```python
from build123d import *

# Parameters (mm, degrees)
BOSS_EXTRUDE1_DEPTH      = 76.2
BOSS_EXTRUDE1_DEPTH_BACK = 76.2
CUT_EXTRUDE1_DEPTH       = 136.619651209
CUT_EXTRUDE1_DEPTH_BACK  = 136.619651209
FILLET1_R                = 3.81
SKETCH14_R               = 2.032
CUT_EXTRUDE8_DEPTH       = 156.372005628
CUT_EXTRUDE9_DEPTH       = 136.355460931
CUT_EXTRUDE9_DEPTH_BACK  = 136.355460931
SKETCH15_W               = 96.731852598
SKETCH15_H               = 147.433285995
SKETCH15_W_2             = 126.258869859
SKETCH15_H_2             = 31.294033563
CUT_EXTRUDE10_DEPTH      = 112.88020808
CUT_EXTRUDE10_DEPTH_BACK = 112.88020808
SKETCH16_R               = 2.127


with BuildPart() as part:
    # Sketch1 → Boss-Extrude1 (new, two sides: drawn at the far end of the back side and taken through both)
    with BuildSketch(Plane.XY.offset(-BOSS_EXTRUDE1_DEPTH_BACK)):
        with BuildLine():
            Line((-6.335258536, -105.245804705), (-12.685258536, -3.645804705))
            ThreePointArc((-12.685258536, -3.645804705), (0.014741464, 8.866413132), (12.714741464, -3.645804705))
            Line((12.714741464, -3.645804705), (6.364741464, -105.245804705))
            ThreePointArc((6.364741464, -105.245804705), (0.014741464, -111.465623147), (-6.335258536, -105.245804705))
        make_face()
    extrude(amount=BOSS_EXTRUDE1_DEPTH + BOSS_EXTRUDE1_DEPTH_BACK)

    # Sketch4 → Cut-Extrude1 (cut, two sides: drawn at the far end of the back side and taken through both)
    with BuildSketch(Plane(origin=(0, 0, 0), x_dir=(0, 0, -1), z_dir=(1, 0, 0)).offset(-CUT_EXTRUDE1_DEPTH_BACK)):
        Polygon((-47.498, -73.524605007), (-47.498, -51.299605007), (47.625, -51.299605007), (47.625, -73.524605007), (76.2, -73.524605007), (76.2, 8.866413132), (-76.2, 8.866413132), (-76.2, -28.682279346), (-76.2, -111.465623147), (-60.198, -111.465623147), (-60.198, -73.524605007), align=None)
    extrude(amount=CUT_EXTRUDE1_DEPTH + CUT_EXTRUDE1_DEPTH_BACK, mode=Mode.SUBTRACT)

    # Fillet1
    fillet1_edges = [part.edges().sort_by_distance(p)[0] for p in [
        (8.347316445, -73.524605007, 53.848),
        (9.736378945, -51.299605007, -0.0635),
        (-9.706896017, -51.299605007, -0.0635),
        (-8.317833517, -73.524605007, 53.848),
        (-8.317833517, -73.524605007, -61.9125),
        (8.347316445, -73.524605007, -61.9125),
    ]]
    fillet(fillet1_edges, radius=FILLET1_R)

    # Sketch14 → Cut-Extrude8 (cut, through all)
    with BuildSketch(Plane(origin=(0, 0, -47.625), x_dir=(-1, 0, 0), z_dir=(0, 0, -1))):
        with Locations((-0.014741464, -61.459605007)):
            Circle(SKETCH14_R)
    extrude(amount=-CUT_EXTRUDE8_DEPTH, mode=Mode.SUBTRACT)

    # Sketch15 → Cut-Extrude9 (cut, two sides: drawn at the far end of the back side and taken through both)
    with BuildSketch(Plane(origin=(0, 0, 0), x_dir=(1, 0, 0), z_dir=(0, 1, 0)).offset(-CUT_EXTRUDE9_DEPTH_BACK)):
        with Locations((-16.666713659, 27.806142998)):
            Rectangle(SKETCH15_W, SKETCH15_H)
        with Locations((-1.903205029, -63.145016782)):
            Rectangle(SKETCH15_W_2, SKETCH15_H_2)
    extrude(amount=CUT_EXTRUDE9_DEPTH + CUT_EXTRUDE9_DEPTH_BACK, mode=Mode.SUBTRACT)

    # Sketch16 → Cut-Extrude10 (cut, two sides: drawn at the far end of the back side and taken through both)
    with BuildSketch(Plane.XY.offset(47.498).offset(-CUT_EXTRUDE10_DEPTH_BACK)):
        with Locations((0.014741464, -106.385623147)):
            Circle(SKETCH16_R)
        with Locations((0.014741464, -83.525623147)):
            Circle(SKETCH16_R)
    extrude(amount=CUT_EXTRUDE10_DEPTH + CUT_EXTRUDE10_DEPTH_BACK, mode=Mode.SUBTRACT)


solid = part.part
```
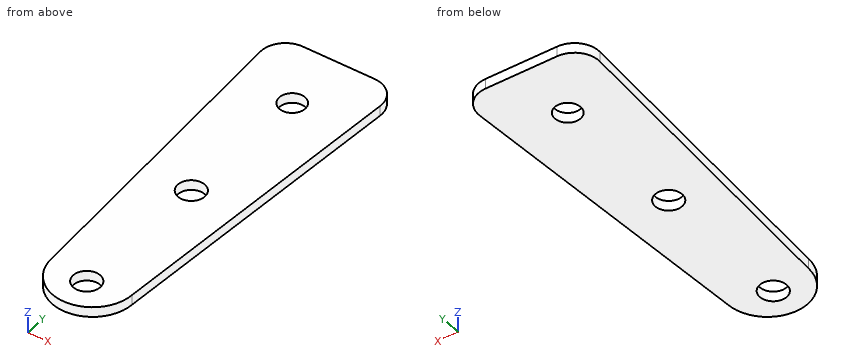
The listing builds one solid part. Answer for the finished solid, in the listing's coordinates (mm). Round coordinates to 2 decimals unless told otherwise and drop trailing zeros. Write each loop counter-clockwise with the first axis right and the second up, starting at its lowest first coordinate (ties: lowest second). Pieces come first, ordered by that corner, then holes. Notation, with made-up numbers: (-1.5, 47) -> (6.5, 47) arc R16 ccw to (6.5, 70) -> close; hole circle Ø7 at (30.25, -0.5). An arc over 180 degrees is marked (long way). Use CSV: the item, a comma, the result in double quotes. Start each with the question number.
(1) This flat-tipped pin is pushed along its axis until it touches: pin 1 (2.5 mm diameter, centred on x = 0.01, y = -106.39, fed in from +Z). Where does it stop, or does it pass through?
(2) Consider L1, parallel to X at y = -83, z = 47.2; L2, parallel to X at y = -105, z = 46.15; L3, parallel to Y at x = -3.5, z = 46.35. Determine where each line is inside the solid, lowest interval first. Write a range as from..to.
(3) Section C-C on y = -69 is taken. Give the vertices of the cut face in (x, z).
(4) Section B-B on z = 46.8 is taken. Give the vertices of the cut face in (x, y).
(5) Section D-D on x = 4.5 is taken. Give the vertices of the cut face in (y, z), then the cut area to 3 significant figures.
(6) Section A-A on x = -1 is taken. Give the vertices of the cut face in (y, z), then the cut area to 3 significant figures.
A:
1,pin 1,"passes through"
2,L1,"x = -7.73..-2.05, 2.08..7.76"
2,L2,"x = -6.35..-1.6, 1.63..6.38"
2,L3,"y = -110.4..-51.3"
3,outline,"(-8.6, 45.91) -> (8.63, 45.91) -> (8.63, 47.5) -> (-8.6, 47.5) -> close"
4,outline,"(-9.45, -55.35) -> (-6.34, -105.25) arc R6.35 ccw to (6.36, -105.25) -> (9.48, -55.35) arc R3.81 ccw to (5.68, -51.3) -> (-5.65, -51.3) arc R3.81 ccw to start; hole circle Ø4.25 at (0.01, -106.39); hole circle Ø4.25 at (0.01, -83.53); hole circle Ø4.06 at (0.01, -61.46)"
5,outline,"(-109.61, 45.91) -> (-51.3, 45.91) -> (-51.3, 47.5) -> (-109.61, 47.5) -> close"
5,area,"92.6 mm²"
6,outline,"(-111.38, 45.91) -> (-108.25, 45.91) -> (-108.25, 47.5) -> (-111.38, 47.5) -> close; (-104.52, 45.91) -> (-85.39, 45.91) -> (-85.39, 47.5) -> (-104.52, 47.5) -> close; (-81.66, 45.91) -> (-63.22, 45.91) -> (-63.22, 47.5) -> (-81.66, 47.5) -> close; (-59.7, 45.91) -> (-51.3, 45.91) -> (-51.3, 47.5) -> (-59.7, 47.5) -> close"
6,area,"77.9 mm²"
